from build123d import *

# Parameters (mm, degrees)
BOTTOM_LEVEL_DEPTH = 5
MID_LEVEL_DEPTH    = 35
GUARD_RAIL_DEPTH   = 100
ROUNDING_R         = 5


with BuildPart() as part:
    # Sketch1 → Bottom level (new body)
    with BuildSketch(Plane(origin=(0, 0, 0), x_dir=(1, 0, 0), z_dir=(0, 1, 0))):
        with BuildLine():
            Line((300, 300), (300, 325))
            ThreePointArc((300, 325), (70.190296114, 229.809703886), (-25, 0))
            Line((-25, 0), (0, 0))
            ThreePointArc((0, 0), (87.867965644, 212.132034356), (300, 300))
        make_face()
    extrude(amount=BOTTOM_LEVEL_DEPTH)

    # Sketch2 → Mid level (add)
    with BuildSketch(Plane(origin=(0, 5, 0), x_dir=(1, 0, 0), z_dir=(0, 1, 0))):
        with BuildLine():
            Line((-25, 0), (-10, 0))
            ThreePointArc((-10, 0), (80.796897832, 219.203102168), (300, 310))
            Line((300, 310), (300, 325))
            ThreePointArc((300, 325), (70.190296114, 229.809703886), (-25, 0))
        make_face()
    extrude(amount=MID_LEVEL_DEPTH)

    # Sketch3 → Guard rail (add)
    with BuildSketch(Plane(origin=(0, 40, 0), x_dir=(1, 0, 0), z_dir=(0, 1, 0))):
        with BuildLine():
            Line((-25, 0), (-20, 0))
            ThreePointArc((-20, 0), (73.72583002, 226.27416998), (300, 320))
            Line((300, 320), (300, 325))
            ThreePointArc((300, 325), (70.190296114, 229.809703886), (-25, 0))
        make_face()
    extrude(amount=GUARD_RAIL_DEPTH)

    # Rounding
    rounding_edges = [part.edges().sort_by_distance(p)[0] for p in [
        (80.796897832, 5, -219.203102168),
        (80.796897832, 40, -219.203102168),
        (73.72583002, 40, -226.27416998),
    ]]
    fillet(rounding_edges, radius=ROUNDING_R - 0.0001)  # a hair under: the kernel refuses the full size


solid = part.part
Input: part model. Units: mm. Frame: model coordinates. A direction names the side the tool comes from. Round coordinates to 2 decimals unless told otherwise and drop trailing zeros. Order: outer loops, then holes, each group sorted by start corner. A loop starts at its lowest first (then second) coordinate and runs counter-clockwise, first axis right, second up. Notation, with made-up numbers: (64, 46.25) - (115, 46.25) arc R32 cw to (115, 72.25) - close; hole circle Ø6 at (74, 50.25). An arc over 180 degrees is marked (long way). Answer as a JSON object with one key per item and string values. Group by question number.
(1) Reachability of faces 1 (the face through (85.55, 2.46, -209.79)), 2 (the face through (78.4, 22.32, -216.78)) from +Z, -Z, +X, -X, +Y, -Y: full face, straight path, thin tool, end or side. Return the list, or none.
(2) Cut plane A-A (y = 21.5). Return loops of the section in (x, z).
(3) Cut plane B-B (y = 108). Return loops of the section in (x, z).
(4) Pin query (flat end, axial travel): P1, Ø6, axis at x = 125.5, y = 56, coming from the -Z side; P2, Ø8, axis at x = 88.5, y = 100.5, coming from the +Z side; P3, Ø1.5, axis at x = 237.5, y = 103, coming from the +Z side. Return the tip coordinate at first contact, or that it passes through.
(5) Material intervals for probe 1 along Y at (x, z) = (77, -201); probe 2 along Y at (x, z) = (101.5, -245); probe 3 along Z at (x, y) = (201.5, 133), sorted ascending. Write a range as from..to.
Here are the results:
{
 "1": {"face 1": "+Z, +X, +Y, -Y", "face 2": "+Z, +X, +Y"},
 "2": {"outline": "(-25, 0) arc R325 ccw to (300, -325) - (300, -310) arc R310 cw to (-10, 0) - close"},
 "3": {"outline": "(-25, 0) arc R325 ccw to (300, -325) - (300, -320) arc R320 cw to (-20, 0) - close"},
 "4": {"P1": "stops at z = -276.07", "P2": "stops at z = -236.56", "P3": "stops at z = -313.69"},
 "5": {"probe 1": "y = 0..5", "probe 2": "y = 0..40.01", "probe 3": "z = -309.71..-304.46"}
}
